Answer from the drawing. Dimensions are ordinates in mm from the lowest x, y and z of the part. A direction names the side the tool comes from. Coordinates: 2 decimals unless noted, no trailing zeros. Loops run counter-clockwise (first coordinate to the right, second up) from the corner with the lowest first, then second, coordinate; pieces in that order, holes last.
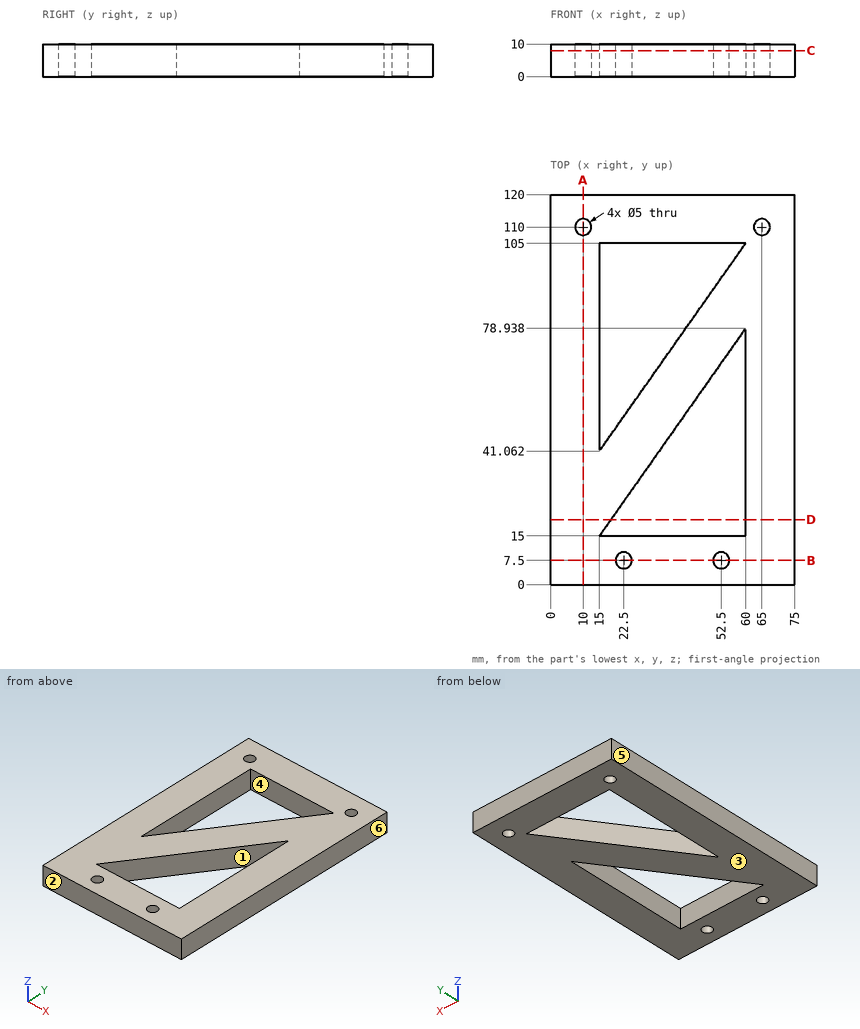
Item 1: A cutting plane is placed at B-B on y = 7.5. Determine the outline of the cut face in (x, z).
Numbers:
outline: (0, 0) - (20, 0) - (20, 10) - (0, 10) - close; (25, 0) - (50, 0) - (50, 10) - (25, 10) - close; (55, 0) - (75, 0) - (75, 10) - (55, 10) - close
Item 2: A cutting plane is placed at D-D on y = 20. Determine the outline of the cut face in (x, z), then the cut area to 3 significant figures.
Numbers:
outline: (0, 0) - (18.52, 0) - (18.52, 10) - (0, 10) - close; (60, 0) - (75, 0) - (75, 10) - (60, 10) - close
area: 335 mm2
Item 3: Determine the mould class of the marked faces 3, 4, 5 and 6 for opening direction X: released by +X, released by -X, zero draft, split by the parting line, or undercut.
Numbers:
face 3: zero draft
face 4: undercut
face 5: released by -X
face 6: released by +X
Item 4: A cutting plane is placed at A-A on x = 10. Determine the outline of the cut face in (y, z), then the cut area to 3 significant figures.
Numbers:
outline: (0, 0) - (107.5, 0) - (107.5, 10) - (0, 10) - close; (112.5, 0) - (120, 0) - (120, 10) - (112.5, 10) - close
area: 1,150 mm2
Item 5: Find the intervals of material crossed by line 1 along Y through (x, z) = (65, 3); line 2 along Y through (x, z) = (29, 7.75); line 3 along Y through (x, z) = (27.5, 4), in increasing order.
Numbers:
line 1: y = 0 to 107.5, 112.5 to 120
line 2: y = 0 to 15, 34.89 to 60.95, 105 to 120
line 3: y = 0 to 15, 32.76 to 58.82, 105 to 120
Item 6: A cutting plane is placed at C-C on z = 8. Determine the outline of the cut face in (x, y).
Numbers:
outline: (0, 0) - (75, 0) - (75, 120) - (0, 120) - close; hole circle Ø5 at (10, 110); hole (15, 15) - (60, 15) - (60, 78.94) - close; hole (15, 41.06) - (60, 105) - (15, 105) - close; hole circle Ø5 at (22.5, 7.5); hole circle Ø5 at (52.5, 7.5); hole circle Ø5 at (65, 110)
Item 7: Which of the six approach directions +Z, -Z, +X, -X, +Y, -Y give full straight-line access (tool end or side, diameter ignored) to the marked faces 1 and 2?
Numbers:
face 1: +Z, -Z
face 2: +Z, -Z, +X, -X, -Y
